```python
from build123d import *

# Parameters (mm, degrees)
F0_W     = 100
F0_H     = 60
F1_DEPTH = 3
F2_W     = 10
F2_H     = 23
F3_DEPTH = 3.001
F4_R     = 3
F5_DEPTH = 3.001


with BuildPart() as f1:
    # F0 (on Top) → F1 (new body)
    with BuildSketch(Plane.XY):
        Rectangle(F0_W, F0_H)
    extrude(amount=F1_DEPTH)

    # F2 (on face) → F3 (cut, through all)
    with BuildSketch(Plane.XY.offset(3)):
        with Locations((-45, 11.5)):
            Rectangle(F2_W, F2_H)
        with Locations((-45, -11.5)):
            Rectangle(F2_W, F2_H)
        with Locations((45, 11.5)):
            Rectangle(F2_W, F2_H)
        with Locations((45, -11.5)):
            Rectangle(F2_W, F2_H)
    extrude(amount=-F3_DEPTH, mode=Mode.SUBTRACT)

    # F4 (on face) → F5 (cut, through all)
    with BuildSketch(Plane.XY.offset(3)):
        with Locations((30, 23)):
            Circle(F4_R)
    extrude(amount=-F5_DEPTH, mode=Mode.SUBTRACT)


solid = f1.part
```
Read the model definition and answer for the solid it produces. Units are mm, in the model's axes. A direction names the side the tool comes from. Round coordinates to 2 decimals unless told otherwise and drop trailing zeros. Write each loop counter-clockwise with the first axis right and the second up, starting at its lowest first coordinate (ties: lowest second). Pieces come first, ordered by that corner, then holes. Notation, with made-up numbers: (-6.5, -33.75) -> (32.5, -33.75) arc R18 ccw to (32.5, -6.75) -> close; hole circle Ø4 at (0.25, -39.5). An arc over 180 degrees is marked (long way). Answer in a Markdown table with one row per item. Add a question column.
1) Find section A-A, the plane x = 30. Determine the outline of the cut face in (y, z).
2) Which of the six approach directions +Z, -Z, +X, -X, +Y, -Y give full straight-line access (tool end or side, diameter ignored) to faces 1 (the face through (-45, 23, 2)), 2 (the face through (-50, -27, 1)), 3 (the face through (45, -23, 2))?
3) Find section C-C, the plane y = -12. Determine the outline of the cut face in (x, z).
4) Determine the mould class of faces 4 (the face through (45, 23, 2)), 5 (the face through (-1, 0, 0)), 6 (the face through (-1, -30, 1)) for opening direction Y: pulls with the +Y half, pulls with the -Y half, needs draft (parallel to the pull), parting line crosses it, or undercut.
5) Given P1, Ø0.9, axis at y = -1.5, z = 1.5, coming from the -X side; P2, Ø0.9, axis at y = 6.5, z = 1.5, coming from the +X side, each flat-ended and moving along its own axis, determine where each tip first touches the part or whether it passes through.
6) Find section B-B, the plane z = 0.95. Determine the outline of the cut face in (x, y).
7) Consider line 1 (Y direction, x = 30, z = 0.6); line 2 (X direction, y = 16, z = 1.4); line 3 (X direction, y = 25.5, z = 1.75). Determine where each line is inside the solid, lowest interval first.
Findings below:
| question | item | result |
|---|---|---|
| 1 | outline | (-30, 0) -> (20, 0) -> (20, 3) -> (-30, 3) -> close; (26, 0) -> (30, 0) -> (30, 3) -> (26, 3) -> close |
| 2 | face 1 | +Z, -Z, -X |
| 2 | face 2 | +Z, -Z, -X, +Y, -Y |
| 2 | face 3 | +Z, -Z, +X |
| 3 | outline | (-40, 0) -> (40, 0) -> (40, 3) -> (-40, 3) -> close |
| 4 | face 4 | undercut |
| 4 | face 5 | needs draft |
| 4 | face 6 | pulls with the -Y half |
| 5 | P1 | x = -40 |
| 5 | P2 | x = 40 |
| 6 | outline | (-50, -30) -> (50, -30) -> (50, -23) -> (40, -23) -> (40, 23) -> (50, 23) -> (50, 30) -> (-50, 30) -> (-50, 23) -> (-40, 23) -> (-40, -23) -> (-50, -23) -> close; hole circle Ø6 at (30, 23) |
| 7 | line 1 | -30 to 20, 26 to 30 |
| 7 | line 2 | -40 to 40 |
| 7 | line 3 | -50 to 28.34, 31.66 to 50 |
